Verification items for the finished model (mm, model axes). Face numbers are marked on the shaded views. A direction names the side the tool comes from. Coordinates: 2 decimals unless noted, no trailing zeros. Loops run counter-clockwise (first coordinate to the right, second up) from the corner with the lowest first, then second, coordinate; pieces in that order, holes last. Notation, with made-up numbers: (-2, -21.5) - (44, -21.5) arc R35 ccw to (44, 14.5) - close; hole circle Ø6 at (-33.75, -1). An arc over 180 degrees is marked (long way). One line per item, written item: value. Start each with the question number.
(1) Section check D-D (y = 8.5). Record the boundary of the cut face in (x, z), plus the area to 3 significant figures.
(2) Set-up check for the marked faces 1, 2 and 3: record each of +Z, -Z, +X, -X, +Y, -Y from which the full face is reachable in a straight line by a thin tool's end or side.
(3) Thickness scan on probe 1 along Y at (x, z) = (10, -0.8); probe 2 along Z at (x, y) = (6.25, 6.5); probe 3 along X at (y, z) = (7, -8). Record the ranges inside material, lowest first. Write a range as [from, to].
(4) Draft check along X on the marked faces 4, 5 and 6. Enter one of: +X half, -X half, draft (parallel to the pull), parting line (faces both ways), or undercut.
(5) Section check C-C (z = -7). Record the boundary of the cut face in (x, y), plus the area to 3 significant figures.
(6) Gauge pin test, flat ends, axial feed: P1, Ø2, axis at x = 10, y = 1.5, coming from the -Z side; P2, Ø5, axis at y = 3.5, z = -10, coming from the +X side; P3, Ø3, axis at y = 4.5, z = -11, coming from the +X side. Record the tip position at first contact, or that the pin passes through.
(7) Section check A-A (x = 8.5). Record the boundary of the cut face in (y, z), plus the area to 3 significant figures.
```python
from build123d import *

# Parameters (mm, degrees)
BOSS_EXTRUDE1_DEPTH = 10
SKETCH2_R           = 1.7
CUT_EXTRUDE1_DEPTH  = 21.615528128
SKETCH3_R           = 1.7
CUT_EXTRUDE2_DEPTH  = 21.615528128
CUT_EXTRUDE3_DEPTH  = 3
CUT_EXTRUDE4_DEPTH  = 3
FILLET1_R           = 5


with BuildPart() as part:
    # Sketch1 → Boss-Extrude1 (new body)
    with BuildSketch(Plane(origin=(0, 0, 0), x_dir=(1, 0, 0), z_dir=(0, 1, 0))):
        Polygon((0, 0), (0, 15), (5, 15), (5, 5), (15, 5), (15, 0), align=None)
    extrude(amount=BOSS_EXTRUDE1_DEPTH)

    # Sketch2 → Cut-Extrude1 (cut, through all)
    with BuildSketch(Plane(origin=(0, 0, -5), x_dir=(-1, 0, 0), z_dir=(0, 0, -1))):
        with Locations((-10, 5)):
            Circle(SKETCH2_R)
    extrude(amount=-CUT_EXTRUDE1_DEPTH, mode=Mode.SUBTRACT)

    # Sketch3 → Cut-Extrude2 (cut, through all)
    with BuildSketch(Plane(origin=(5, 0, 0), x_dir=(0, 0, -1), z_dir=(1, 0, 0))):
        with Locations((10, 5)):
            Circle(SKETCH3_R)
    extrude(amount=-CUT_EXTRUDE2_DEPTH, mode=Mode.SUBTRACT)

    # Sketch4 → Cut-Extrude3 (cut)
    with BuildSketch(Plane(origin=(5, 0, 0), x_dir=(0, 0, -1), z_dir=(1, 0, 0))):
        Polygon((13.464101615, 5), (11.732050808, 8), (8.267949192, 8), (6.535898385, 5), (8.267949192, 2), (11.732050808, 2), align=None)
    extrude(amount=-CUT_EXTRUDE3_DEPTH, mode=Mode.SUBTRACT)

    # Sketch5 → Cut-Extrude4 (cut)
    with BuildSketch(Plane(origin=(0, 0, -5), x_dir=(-1, 0, 0), z_dir=(0, 0, -1))):
        Polygon((-6.535898385, 5), (-8.267949192, 8), (-11.732050808, 8), (-13.464101615, 5), (-11.732050808, 2), (-8.267949192, 2), align=None)
    extrude(amount=-CUT_EXTRUDE4_DEPTH, mode=Mode.SUBTRACT)

    # Fillet1
    fillet1_edges = [part.edges().sort_by_distance(p)[0] for p in [
        (0, 5, 0),
        (15, 10, -2.5),
        (15, 0, -2.5),
        (2.5, 0, -15),
        (2.5, 10, -15),
    ]]
    fillet(fillet1_edges, radius=FILLET1_R - 0.0001)  # a hair under: the kernel refuses the full size


solid = part.part
```
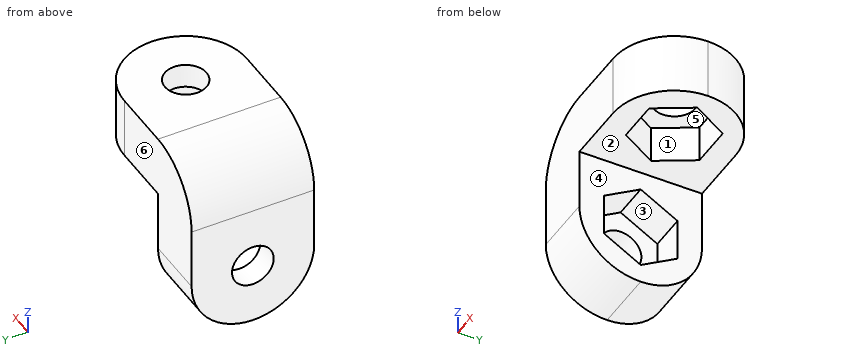
Responses:
1. outline: (0, -13.57) - (5, -13.57) - (5, -5) - (13.57, -5) - (13.57, 0) - (5, 0) arc R5 ccw to (0, -5) - close
1. area: 105 mm²
2. face 1: -Z
2. face 2: -Z, +X, +Y, -Y
2. face 3: +X
3. probe 1: y = [0, 3.3], [6.7, 10]
3. probe 2: z = [-5, 0]
3. probe 3: x = [0, 2]
4. face 4: +X half
4. face 5: undercut
4. face 6: draft
5. outline: (0, 0) - (5, 0) - (5, 4.2) - (2, 4.2) - (2, 5.8) - (5, 5.8) - (5, 10) - (0, 10) - close
5. area: 45.2 mm²
6. P1: stops at z = -5
6. P2: stops at x = 5
6. P3: stops at x = 2
7. outline: (0, -5) - (2, -5) - (2, -2) - (4.2, -2) - (4.2, 0) - (0, 0) - close; (5.8, -2) - (8, -2) - (8, -5) - (10, -5) - (10, 0) - (5.8, 0) - close
7. area: 28.8 mm²
